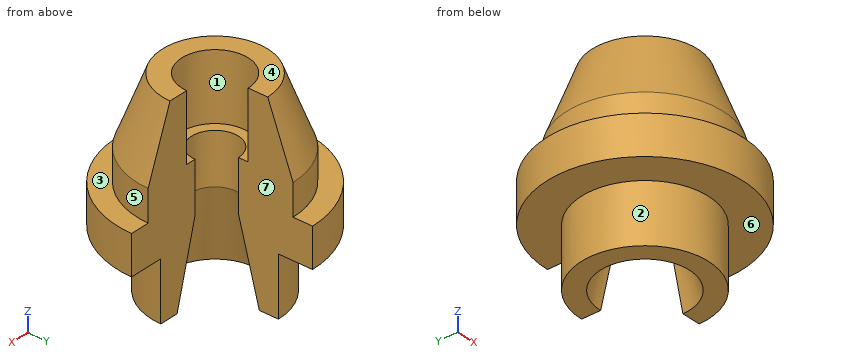
```python
from build123d import *

# Parameters (mm, degrees)
REVOLVE1_ANGLE = 270


with BuildPart() as part:
    # Sketch1 → Revolve1 (revolve)
    with BuildSketch(Plane(origin=(0, 0, 0), x_dir=(0, 0, -1), z_dir=(1, 0, 0))):
        Polygon((0, 0), (0, 27), (34, 40), (50, 40), (50, 50), (70, 50), (70, 32.5), (100, 32.5), (100, 0), align=None)
    revolve(axis=Axis((0, 0, -100), (0, 0, 1)), revolution_arc=REVOLVE1_ANGLE)

    # Sketch3 → Cut-Revolve1 (revolve, cut)
    with BuildSketch(Plane(origin=(0, 0, 0), x_dir=(0, 0, -1), z_dir=(1, 0, 0))):
        Polygon((0, 17), (0, 0), (100, 0), (100, 22.717967697), (60, 12), (34, 12), (34, 17), align=None)
    revolve(axis=Axis((0, 0, 0), (0, 0, -1)), mode=Mode.SUBTRACT)


solid = part.part
```
Source: CAD feature listing. Evaluate the final solid. Frame: model axes, mm. Face numbers are marked on the shaded views. A direction names the side the tool comes from. Give positions to 0.01 mm unless a question says otherwise; leave off trailing zeros. Loops run counter-clockwise (first coordinate to the right, second up) from the corner with the lowest first, then second, coordinate; pieces in that order, holes last. Notation, with made-up numbers: (57.25, -26.5) -> (91.25, -26.5) arc R16 cw to (91.25, 3.5) -> close; hole circle Ø5 at (88, -18.5). An arc over 180 degrees is marked (long way). Put each result on its own line as item: value. Start each with the question number.
1) Cut plane B-B (y = -41.5). Return loops of the section in (x, z).
2) Contact query for flat-ended pins moving along their axis: P1, Ø4, axis at x = 28.5, z = -32, coming from the -Y side; P2, Ø19, axis at x = 31, z = -56, coming from the +Y side; P3, Ø2, axis at y = 30.5, z = -41.5, coming from the +X side. Output: stop coordinate, or through.
3) Reachability of the marked faces 4, 5, 6 and 7 from +Z, -Z, +X, -X, +Y, -Y: full face, straight path, thin tool, end or side. Return the list, or none.
4) Material intervals for probe 1 along Z at (x, y) = (-42, 1.5); probe 2 along Y at (x, z) = (-14, -11); probe 3 along Y at (x, z) = (-10, -63), sorted ascending.
5) Cut plane A-A (z = -43.5). Return loops of the section in (x, y).
6) Draft query along Y for the marked faces 1, 2 and 3. Return one class per face: released by +Y, released by -Y, zero draft, split by the parting line, or undercut.
Results are:
1. outline: (-27.89, -70) -> (27.89, -70) -> (27.89, -50) -> (-27.89, -50) -> close
2. P1: stops at y = -29.21
2. P2: stops at y = 0
2. P3: stops at x = 0
3. face 4: +Z, +X, -X, +Y, -Y
3. face 5: +Z
3. face 6: -Z
3. face 7: +Z, -Z, +X, +Y
4. probe 1: z = -70 to -50
4. probe 2: y = -27.89 to -9.64, 9.64 to 27.89
4. probe 3: y = -48.99 to -8, 8 to 48.99
5. outline: (0, 12) -> (0, 40) arc R40 ccw (long way) to (40, 0) -> (12, 0) arc R12 cw (long way) to start
6. face 1: undercut
6. face 2: split by the parting line
6. face 3: zero draft
